```python
from build123d import *

# Parameters (mm, degrees)
F0_W      = 15
F0_H      = 18
F1_DEPTH  = 4.4
F2_R      = 2
F3_SIZE2  = 9.99999
F3_SIZE   = 17.99999
F4_R      = 2
F6_W      = 8
F6_H      = 4.4
F6_W_2    = 15
F7_DEPTH  = 4
F8_DEPTH  = 4
F9_SIZE2  = 15
F9_SIZE   = 4
F10_DEPTH = 4.4
F11_R     = 1
F12_DEPTH = 4.4


# Not quite as in the source:
# - a fillet or chamfer is up to 0.001 mm smaller than in the source, because OpenCascade refuses the exact size


with BuildPart() as f1:
    # F0 (on Top) → F1 (new body)
    with BuildSketch(Plane.XY):
        with Locations((7.5, 9)):
            Rectangle(F0_W, F0_H)
    extrude(amount=F1_DEPTH)

    # F2
    f2_edges = [f1.edges().sort_by_distance(p)[0] for p in [
        (0, 0, 2.2),
    ]]
    fillet(f2_edges, radius=F2_R)

    # F3 (size 18 and 10 in the source; OpenCascade refuses exactly that, so slightly less here)
    f3_edges = [f1.edges().sort_by_distance(p)[0] for p in [
        (15, 0, 2.2),
    ]]
    f3_side = f1.faces().sort_by_distance((15, 9, 2.2))[0]
    chamfer(f3_edges, length=F3_SIZE, length2=F3_SIZE2, reference=f3_side)

    # F4
    f4_edges = [f1.edges().sort_by_distance(p)[0] for p in [
        (5.00001, 0, 2.2),
    ]]
    fillet(f4_edges, radius=F4_R)

    # F6 (on face) → F7 (join)
    with BuildSketch(Plane(origin=(0, 18, 0), x_dir=(-1, 0, 0), z_dir=(0, 1, 0))):
        with Locations((4, 2.2)):
            Rectangle(F6_W, F6_H)
        with Locations((-7.5, 2.2)):
            Rectangle(F6_W_2, F6_H)
    extrude(amount=F7_DEPTH)

    # F8 (add): a face of the model
    f8_faces = [f1.faces().sort_by_distance(p)[0] for p in [
        (3.5, 22, 2.2),
    ]]
    extrude(f8_faces, amount=F8_DEPTH)

    # F9
    f9_edges = [f1.edges().sort_by_distance(p)[0] for p in [
        (-8, 26, 2.2),
    ]]
    f9_side = f1.faces().sort_by_distance((-8, 22, 2.2))[0]
    chamfer(f9_edges, length=F9_SIZE, length2=F9_SIZE2, reference=f9_side)

    # F5 (on face) → F10 (cut)
    with BuildSketch(Plane(origin=(0, 0, 0), x_dir=(1, 0, 0), z_dir=(0, 0, -1))):
        with BuildLine():
            ThreePointArc((2, -3), (3, -4), (4, -3))
            ThreePointArc((4, -3), (3, -2), (2, -3))
        make_face()
    extrude(amount=-F10_DEPTH, mode=Mode.SUBTRACT)

    # F11 (on face) → F12 (cut)
    with BuildSketch(Plane(origin=(0, 0, 0), x_dir=(1, 0, 0), z_dir=(0, 0, -1))):
        with Locations((11.6287460551, -21.6625984758)):
            Circle(F11_R)
    extrude(amount=-F12_DEPTH, mode=Mode.SUBTRACT)


solid = f1.part
```
Geometry: final body of the model. Coordinates: model frame, mm. A direction names the side the tool comes from. Round coordinates to 2 decimals unless told otherwise and drop trailing zeros. Order: outer loops, then holes, each group sorted by start corner. A loop starts at its lowest first (then second) coordinate and runs counter-clockwise, first axis right, second up. Notation, with made-up numbers: (20.5, 20.25) - (25.5, 20.25) arc R21 ccw to (25.5, 48.25) - close; hole circle Ø2 at (12.25, -33). An arc over 180 degrees is marked (long way). Use CSV: the item, a comma, the result in double quotes. Start each with the question number.
Q1. Section query D-D (y = 23). Return loops of the section in (x, z).
Q2. Mould query, pull axis X, two halves, no side actions, for faces 1 (the face through (-0.39, 24.03, 2.17)), 2 (the face through (11.41, 22.64, 2.17)), 3 (the face through (15, 22, 2)). Classes: +X half, -X half, draft (parallel to the pull), parting line (faces both ways), or undercut.
Q3. Section query A-A (y = 3). Return loops of the section in (x, z), and give its area (3 significant figures).
Q4. Access query for faces 4 (the face through (0, 10, 2)), 5 (the face through (11, 26, 2)). Directions: +Z, -Z, +X, -X, +Y, -Y. A direction counts if a zero-diameter tool reaches every point of the face in a straight line with its end or side. Return the directions, or none.
Q5. Section query C-C (z = 1.8). Return loops of the section in (x, y).
Q6. Material intervals for line 1 along Y through (x, z) = (3, 1.65); line 2 along Y through (x, z) = (2.5, 4.05); line 3 along Y through (x, z) = (-7, 3.9), sorted ascending. Write a range as from..to.
Q7. Section query B-B (x = 3). Return loops of the section in (y, z).
Q8. First-contact query: pin 1 (10 mm diameter, centred on x = -2.5, y = 4.5, fed in from -Z); pin 2 (1.3 mm diameter, centred on x = -5, z = 3, fed in from -Y). Flat tips, straight axial feed; report the tip coordinate or a pass-through.
Result set:
1,outline,"(-4.25, 0) - (15, 0) - (15, 4.4) - (-4.25, 4.4) - close"
2,face 1,"-X half"
2,face 2,"undercut"
2,face 3,"+X half"
3,outline,"(0, 0) - (2, 0) - (2, 4.4) - (0, 4.4) - close; (4, 0) - (6.67, 0) - (6.67, 4.4) - (4, 4.4) - close"
3,area,"20.5 mm2"
4,face 4,"+Z, -Z, -X, -Y"
4,face 5,"+Z, -Z, +X, -X, +Y"
5,outline,"(-8, 18) - (0, 18) - (0, 2) arc R2 ccw to (2, 0) - (3.82, 0) arc R2 ccw to (5.57, 1.03) - (15, 18) - (15, 26) - (7, 26) - (-8, 22) - close; hole circle Ø2 at (3, 3); hole circle Ø2 at (11.63, 21.66)"
6,line 1,"y = 0..2, 4..24.93"
6,line 2,"y = 0..2.13, 3.87..24.8"
6,line 3,"y = 18..22.27"
7,outline,"(0, 0) - (2, 0) - (2, 4.4) - (0, 4.4) - close; (4, 0) - (24.93, 0) - (24.93, 4.4) - (4, 4.4) - close"
8,pin 1,"stops at z = 0"
8,pin 2,"stops at y = 18"
